from build123d import *

# Parameters (mm, degrees)
SKETCH1_W           = 79.6544
SKETCH1_H           = 46.228
BOSS_EXTRUDE1_DEPTH = 2.54
SKETCH2_W           = 2.54
SKETCH2_H           = 11.176
BOSS_EXTRUDE2_DEPTH = 79.6544
SKETCH3_R           = 2.1971
CUT_EXTRUDE1_DEPTH  = 94.112727805
SKETCH4_R           = 2.794
BOSS_EXTRUDE3_DEPTH = 1.905
FILLET1_R           = 10.16
FILLET2_R           = 1.27
SKETCH5_R           = 1.524
BOSS_EXTRUDE4_DEPTH = 40.005
SKETCH6_R           = 1.60655
CUT_EXTRUDE2_DEPTH  = 2.54
CHAMFER1_SIZE       = 2.54


with BuildPart() as part:
    # Sketch1 → Boss-Extrude1 (new body)
    with BuildSketch(Plane(origin=(0, 0, 0), x_dir=(1, 0, 0), z_dir=(0, 1, 0))):
        with Locations((39.8272, 23.114)):
            Rectangle(SKETCH1_W, SKETCH1_H)
    extrude(amount=BOSS_EXTRUDE1_DEPTH)

    # Sketch2 → Boss-Extrude2 (add)
    with BuildSketch(Plane(origin=(79.6544, 0, 0), x_dir=(0, 0, -1), z_dir=(1, 0, 0))):
        with Locations((1.27, 8.128)):
            Rectangle(SKETCH2_W, SKETCH2_H)
    extrude(amount=-BOSS_EXTRUDE2_DEPTH)

    # Sketch3 → Cut-Extrude1 (cut, through all)
    with BuildSketch(Plane.XY):
        with Locations((10.9347, 5.1689)):
            Circle(SKETCH3_R)
        with Locations((29.9847, 5.1689)):
            Circle(SKETCH3_R)
        with Locations((49.0347, 5.1689)):
            Circle(SKETCH3_R)
        with Locations((68.0847, 5.1689)):
            Circle(SKETCH3_R)
    extrude(amount=-CUT_EXTRUDE1_DEPTH, mode=Mode.SUBTRACT)

    # Sketch4 → Boss-Extrude3 (add)
    with BuildSketch(Plane.XY):
        with Locations(Location((13.208, 10.922, 0), (0, 0, 90))):
            Circle(SKETCH4_R)
        with Locations(Location((32.766, 10.922, 0), (0, 0, 90))):
            Circle(SKETCH4_R)
        with Locations(Location((45.974, 10.922, 0), (0, 0, 90))):
            Circle(SKETCH4_R)
        with Locations(Location((66.04, 10.922, 0), (0, 0, 90))):
            Circle(SKETCH4_R)
    extrude(amount=BOSS_EXTRUDE3_DEPTH)

    # Fillet1
    fillet1_edges = [part.edges().sort_by_distance(p)[0] for p in [
        (79.6544, 13.716, -1.27),
        (0, 13.716, -1.27),
    ]]
    fillet(fillet1_edges, radius=FILLET1_R)

    # Fillet2
    fillet2_edges = [part.edges().sort_by_distance(p)[0] for p in [
        (13.208, 8.128, 1.905),
        (32.766, 8.128, 1.905),
        (45.974, 8.128, 1.905),
        (66.04, 8.128, 1.905),
    ]]
    fillet(fillet2_edges, radius=FILLET2_R)

    # Sketch5 → Boss-Extrude4 (add)
    with BuildSketch(Plane(origin=(0, 0, -2.54), x_dir=(-1, 0, 0), z_dir=(0, 0, -1))):
        with Locations(Location((-66.04, 10.922, 0), (0, 0, 180))):
            Circle(SKETCH5_R)
        with Locations(Location((-45.974, 10.922, 0), (0, 0, 180))):
            Circle(SKETCH5_R)
        with Locations(Location((-32.766, 10.922, 0), (0, 0, 180))):
            Circle(SKETCH5_R)
        with Locations(Location((-13.208, 10.922, 0), (0, 0, 180))):
            Circle(SKETCH5_R)
    extrude(amount=BOSS_EXTRUDE4_DEPTH)

    # Sketch6 → Cut-Extrude2 (cut)
    with BuildSketch(Plane.XZ):
        with BuildLine():
            ThreePointArc((41.43375, -8.59155), (40.963202399, -7.455547601), (39.8272, -6.985))
            Line((39.8272, -6.985), (39.8272, -8.59155))
            Line((39.8272, -8.59155), (38.22065, -8.59155))
            ThreePointArc((38.22065, -8.59155), (39.8272, -10.1981), (41.43375, -8.59155))
        make_face()
        with BuildLine():
            Line((39.8272, -8.59155), (39.8272, -6.985))
            ThreePointArc((39.8272, -6.985), (38.691197601, -7.455547601), (38.22065, -8.59155))
            Line((38.22065, -8.59155), (39.8272, -8.59155))
        make_face()
        with Locations(Location((57.6072, -8.59155, 0), (0, 0, 270))):
            Circle(SKETCH6_R)
        with Locations(Location((22.0472, -8.59155, 0), (0, 0, 270))):
            Circle(SKETCH6_R)
        with Locations(Location((4.2672, -8.59155, 0), (0, 0, 270))):
            Circle(SKETCH6_R)
        with Locations(Location((75.3872, -8.59155, 0), (0, 0, 270))):
            Circle(SKETCH6_R)
    extrude(amount=-CUT_EXTRUDE2_DEPTH, mode=Mode.SUBTRACT)

    # Chamfer1
    chamfer1_edges = [part.edges().sort_by_distance(p)[0] for p in [
        (57.6072, 2.54, -6.985),
        (22.0472, 2.54, -6.985),
        (4.2672, 2.54, -6.985),
        (75.3872, 2.54, -6.985),
        (38.22065, 2.54, -8.59155),
    ]]
    chamfer(chamfer1_edges, length=CHAMFER1_SIZE - 0.0001)  # a hair under: the kernel refuses the full size


solid = part.part
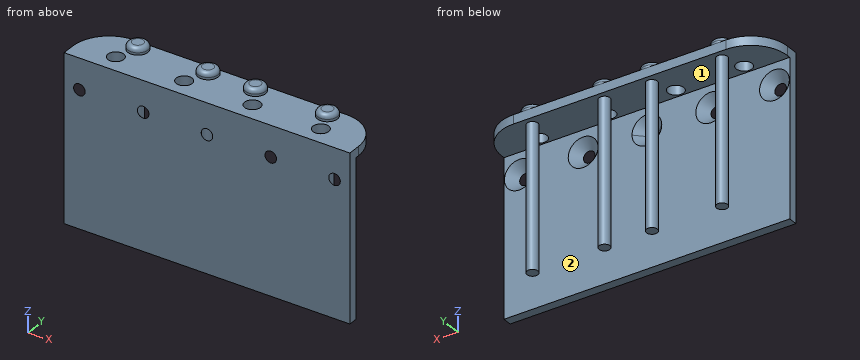
The listing builds one solid part. Answer for the finished solid, in the listing's coordinates (mm). Face numbers are marked on the shaded views. Give positions to 0.01 mm unless a question says otherwise; leave off trailing zeros. Write each loop counter-clockwise with the first axis right and the second up, starting at its lowest first coordinate (ties: lowest second). Pieces come first, ordered by that corner, then holes. Notation, with made-up numbers: (6.5, 53.5) -> (32.5, 53.5) arc R19 cw to (32.5, 64.5) -> close; hole circle Ø6 at (29, 5.25). An arc over 180 degrees is marked (long way). One line per question, with ' | ' between items. Start each with the question number.
1. Section A-A (z = -24) is taken. Determine the outline of the cut face in (x, y), plus the area to 3 significant figures.
2. Given pin 1 Ø5 at (x, z) = (32, -40.5) entering from +Y; pin 2 Ø5 at (y, z) = (10, -13.5) entering from -X; pin 3 Ø5.5 at (x, y) = (29.98, 5.17) entering from +Z, each flat-ended and moving along its own axis, determine where each tip first touches the part or whether it passes through.
3. Section C-C (y = 6) is taken. Determine the outline of the cut face in (x, z), plus the area to 3 significant figures.
4. Find the intervals of material crossed by probe 1 along X at (y, z) = (11.75, -38); probe 2 along Z at (x, y) = (7, 1); probe 3 along Z at (x, y) = (15, 7.25), in increasing order.
5. For a pull along X with two mould halves and no side action, classify the marked faces 1 and 2 as pulls with the +X half, pulls with the -X half, needs draft (parallel to the pull), parting line crosses it, or undercut.
6. Section B-B (x = 52) is taken. Determine the outline of the cut face in (y, z).
Response values:
1) outline: (0, 0) -> (79.65, 0) -> (79.65, 2.54) -> (0, 2.54) -> close; circle Ø3.05 at (13.21, 10.92); circle Ø3.05 at (32.77, 10.92); circle Ø3.05 at (45.97, 10.92); circle Ø3.05 at (66.04, 10.92) | area: 232 mm2
2) pin 1: y = 12.45 | pin 2: x = 11.68 | pin 3: z = 0
3) outline: (0.3, -2.54) -> (8.9, -2.54) -> (8.9, 0) -> (0.3, 0) -> close; (12.97, -2.54) -> (27.95, -2.54) -> (27.95, 0) -> (12.97, 0) -> close; (32.02, -2.54) -> (47, -2.54) -> (47, 0) -> (32.02, 0) -> close; (51.07, -2.54) -> (66.05, -2.54) -> (66.05, 0) -> (51.07, 0) -> close; (70.12, -2.54) -> (79.36, -2.54) -> (79.36, 0) -> (70.12, 0) -> close | area: 159 mm2
4) probe 1: 11.93 to 14.49, 31.49 to 34.05, 44.69 to 47.25, 64.76 to 67.32 | probe 2: -46.23 to 0 | probe 3: -2.54 to 0
5) face 1: undercut | face 2: needs draft
6) outline: (0, -46.23) -> (2.54, -46.23) -> (2.54, -2.54) -> (13.72, -2.54) -> (13.72, 0) -> (0, 0) -> close
